Source: CAD feature listing. Evaluate the final solid. Frame: model axes, mm. A direction names the side the tool comes from. Give positions to 0.01 mm unless a question says otherwise; leave off trailing zeros. Order: outer loops, then holes, each group sorted by start corner. A loop starts at its lowest first (then second) coordinate and runs counter-clockwise, first axis right, second up. Notation, with made-up numbers: M 24.5,24 L 37.5,24 A32 ccw 37.5,58 Z; hole C -9.75,35 d9. An arc over 180 degrees is marked long. Answer as a JSON object with one key per item and string values. Group by question number.
1. Section query C-C (z = 40). Output: boundary loops of the cut face in (x, y).
2. Set-up query: faces 1 (the flat face through (-8, -0.5, 31)), 2 (the flat face through (-64, 6, 44.5)), 3 (the flat face through (-17, 3, 55)), 4 (the flat face through (-2, 3, 11.5)), 5 (the flat face through (-32.7, 7, 53)). Return all of +Z, -Z, +X, -X, +Y, -Y with unobstructed straight access to the full face (end or side cutting, diameter ignored); none if empty.
3. Section query A-A (x = -25.5). Output: boundary loops of the cut face in (y, z).
4. Section query B-B (x = -7). Output: boundary loops of the cut face in (y, z), plus the area to 4 significant figures.
5. Section query D-D (z = 58). Output: boundary loops of the cut face in (x, y).
6. Material intervals for L1, parallel to X at y = 1.1, z = 18; L2, parallel to Z at x = -80, y = 0.5; L3, parallel to Z at x = -85.5, y = 3.75, sorted ascending. Write a range as [from, to].
7. Pull-direction query (X, two-part tool) for faces 6 (the flat face through (-2, 3, 4)), 7 (the flat face through (-12.5, -1.5, 40)), 8 (the flat face through (-50, 4, 5)); classes: +X half, -X half, draft (parallel to the pull), parting line (faces both ways), or undercut.
8. Pin query (flat end, axial travel): P1, Ø3, axis at x = -47, z = 50, coming from the +Y side; P2, Ø5.5, axis at x = -64.5, y = 9.5, coming from the +Z side; P3, Ø1.5, axis at x = -26, y = 9.5, coming from the +Z side; P4, Ø4.5, axis at y = 3, z = 3, coming from the +X side. Return the tip coordinate at first contact, or that it passes through.
Autodesk Inventor part; units mm, degrees
ref_plane "YZ Plane" through (0, 0, 0) normal (1, 0, 0) x (0, 1, 0)
ref_plane "XZ Plane" through (0, 0, 0) normal (0, 1, 0) x (-1, 0, 0)
ref_plane "XY Plane" through (0, 0, 0) normal (0, 0, 1) x (1, 0, 0)
sketch "Skizze1" plane through (0, 0, 0) normal (0, 1, 0) x (-1, 0, 0)
  line L0 (0, 0) -> (85, 0)
  line L1 (85, 0) -> (85, 56)
  line L2 (85, 56) -> (0, 56)
  line L3 (0, 56) -> (0, 0)
  dimension "d0" = 85
  dimension "d1" = 56
extrude "Extrusion1" add sketch "Skizze1" along normal blind 1.5
sketch "Skizze2" plane through (0, 1.5, 0) normal (0, 1, 0) x (1, 0, 0)
  line L0 (0, 0) -> (-85, 0)
  line L1 (-86, -17.2) -> (-65, -17.2)
  line L2 (-65, -17.2) -> (-65, -1.2)
  line L3 (-65, -1.2) -> (-86, -1.2)
  line L4 (-86, -1.2) -> (-86, -17.2)
  line L5 (-85, 0) -> (-85, -56)
  dimension "d4" = 21
  dimension "d5" = 16
  dimension "d6" = 1.2
  dimension "d84" = 1
extrude "Extrusion2" add sketch "Skizze2" along normal blind 13.4
sketch "Skizze3" plane through (0, 1.5, 0) normal (0, 1, 0) x (1, 0, 0)
  line L0 (-85, -17.2) -> (-85, -56)
  line L1 (-92.7, -24) -> (-75.5, -24)
  line L2 (-75.5, -24) -> (-75.5, -37.2)
  line L3 (-75.5, -37.2) -> (-92.7, -37.2)
  line L4 (-92.7, -37.2) -> (-92.7, -24)
  line L5 (-85, -56) -> (0, -56)
  dimension "d9" = 7.7
  dimension "d10" = 17.2
  dimension "d11" = 13.2
  dimension "d85" = 18.8
extrude "Extrusion3" add sketch "Skizze3" along normal blind 16
sketch "Skizze4" plane through (0, 1.5, 0) normal (0, 1, 0) x (1, 0, 0)
  line L0 (0, 0) -> (-85, 0)
  line L1 (-65, -1.2) -> (-65, -17.2)
  line L2 (-50, 1) -> (-35, 1)
  line L3 (-35, 1) -> (-35, -10.8)
  line L4 (-35, -10.8) -> (-50, -10.8)
  line L5 (-50, -10.8) -> (-50, 1)
  dimension "d15" = 1
  dimension "d16" = 15
  dimension "d17" = 11.8
  dimension "d18" = 15
extrude "Extrusion4" add sketch "Skizze4" along normal blind 5.5
sketch "Skizze5" plane through (0, 1.5, 0) normal (0, 1, 0) x (1, 0, 0)
  line L0 (-85, -37.2) -> (-85, -56)
  line L1 (-85, -56) -> (0, -56)
  line L2 (-58.5, -44.5) -> (-70.5, -44.5)
  line L3 (-70.5, -44.5) -> (-70.5, -56)
  line L4 (-70.5, -56) -> (-58.5, -56)
  line L5 (-58.5, -56) -> (-58.5, -44.5)
  line L6 (-70.5, -56) -> (-58.5, -56)
  dimension "d21" = 11.5
  dimension "d22" = 12
  dimension "d23" = 14.5
extrude "Extrusion5" add sketch "Skizze5" along normal blind 10
sketch "Skizze6" plane through (-85, 0, 56) normal (0, 0, 1) x (1, 0, 0)
  line L0 (14.5, 11.5) -> (26.5, 11.5)
  circle A0 centre (20.5, 8) radius 3.5
  dimension "d26" = 7
  dimension "d27" = 3.5
extrude "Extrusion6" add sketch "Skizze6" along normal blind 3.5
sketch "Skizze7" plane through (0, 1.5, 0) normal (0, 1, 0) x (1, 0, 0)
  line L0 (-58.5, -44.5) -> (-58.5, -56)
  line L1 (-58.5, -56) -> (0, -56)
  line L2 (-51, -43.5) -> (-41, -43.5)
  line L3 (-41, -43.5) -> (-41, -53.5)
  line L4 (-41, -53.5) -> (-51, -53.5)
  line L5 (-51, -53.5) -> (-51, -43.5)
  dimension "d30" = 10
  dimension "d31" = 10
  dimension "d32" = 2.5
  dimension "d33" = 7.5
extrude "Extrusion7" add sketch "Skizze7" along normal blind 10.2
sketch "Skizze8" plane through (-51, 1.5, 53.5) normal (0, 0, 1) x (1, 0, 0)
  line L0 (0, 10.2) -> (10, 10.2)
  circle A0 centre (5, 6.2) radius 4
  point P0 (51, -1.5)
  dimension "d36" = 8
  dimension "d37" = 0
extrude "Extrusion8" add sketch "Skizze8" along normal blind 9
sketch "Skizze9" plane through (0, 1.5, 0) normal (0, 1, 0) x (1, 0, 0)
  line L0 (-58.5, -56) -> (0, -56)
  line L1 (0, -56) -> (0, 0)
  line L2 (-1, -55) -> (-33.7, -55)
  line L3 (-33.7, -55) -> (-33.7, -50)
  line L4 (-33.7, -50) -> (-1, -50)
  line L5 (-1, -50) -> (-1, -55)
  dimension "d40" = 32.7
  dimension "d41" = 5
  dimension "d42" = 1
  dimension "d43" = 1
extrude "Extrusion9" add sketch "Skizze9" along normal blind 2.5
sketch "Skizze10" plane through (0, 4, 0) normal (0, 1, 0) x (1, 0, 0)
  line L0 (-33.7, -55) -> (-1, -55)
  line L1 (-1, -55) -> (-1, -50)
  line L2 (-1, -50) -> (-33.7, -50)
  line L3 (-33.7, -50) -> (-33.7, -55)
  line L4 (-32.7, -51) -> (-2, -51)
  line L5 (-2, -51) -> (-2, -54)
  line L6 (-2, -54) -> (-32.7, -54)
  line L7 (-32.7, -54) -> (-32.7, -51)
  point P0 (0, 0)
  dimension "d50" = 1
  dimension "d51" = 1
  dimension "d52" = 1
  dimension "d53" = 1
extrude "Extrusion10" add sketch "Skizze10" along normal blind 6 contours L4 L5 L6 L7
sketch "Skizze11" plane through (0, 1.5, 0) normal (0, 1, 0) x (1, 0, 0)
  line L0 (0, -56) -> (0, 0)
  line L1 (0, 0) -> (-35, 0)
  line L2 (1, -4) -> (-4.6, -4)
  line L3 (-4.6, -4) -> (-4.6, -11.5)
  line L4 (-4.6, -11.5) -> (1, -11.5)
  line L5 (1, -11.5) -> (1, -4)
  dimension "d56" = 1
  dimension "d57" = 7.5
  dimension "d58" = 5.6
  dimension "d59" = 4
extrude "Extrusion11" add sketch "Skizze11" along normal blind 3
sketch "Skizze12" plane through (0, 0, 0) normal (0, -1, 0) x (1, 0, 0)
  line L0 (0, 0) -> (-85, 0)
  line L1 (0, 56) -> (0, 0)
  line L2 (-1, 43.5) -> (-18, 43.5)
  line L3 (-18, 43.5) -> (-18, 15.5)
  line L4 (-18, 15.5) -> (-1, 15.5)
  line L5 (-1, 15.5) -> (-1, 43.5)
  dimension "d62" = 15.5
  dimension "d63" = 17
  dimension "d64" = 28
  dimension "d65" = 1
extrude "Extrusion12" add sketch "Skizze12" along normal blind 0.5
sketch "Skizze13" plane through (0, -0.5, 0) normal (0, -1, 0) x (1, 0, 0)
  line L0 (-1, 43.5) -> (-18, 43.5)
  line L1 (-18, 43.5) -> (-18, 15.5)
  line L2 (-18, 15.5) -> (-1, 15.5)
  line L3 (-1, 15.5) -> (-1, 43.5)
  line L4 (-15, 42.5) -> (-1, 42.5)
  line L5 (-1, 42.5) -> (-1, 18.5)
  line L6 (-1, 18.5) -> (-15, 18.5)
  line L7 (-15, 18.5) -> (-15, 42.5)
  line L8 (-15, 37.5) -> (-10, 42.5)
  line L9 (-15, 37.5) -> (-7.9289, 37.5) construction
  point P0 (0, 0)
  dimension "d69" = 24
  dimension "d70" = 3
  dimension "d71" = 3
  dimension "d72" = 45
  dimension "d73" = 19
extrude "Extrusion13" add sketch "Skizze13" along normal blind 2 contours L3 L4 L7 L6 L2 L1 L0 | L8 L7 L4
sketch "Skizze14" plane through (0, 1.5, 0) normal (0, 1, 0) x (1, 0, 0)
  line L0 (0, 0) -> (-35, 0)
  line L1 (-85, -37.2) -> (-85, -56)
  line L2 (-85, -56) -> (-70.5, -56)
  line L3 (0, -56) -> (0, -11.5)
  circle A0 centre (-25.5, -18) radius 1.45
  circle A1 centre (-80, -43.5) radius 1.45
  dimension "d76" = 2.9
  dimension "d77" = 25.5
  dimension "d78" = 18
  dimension "d79" = 2.9
  dimension "d80" = 5
  dimension "d81" = 12.5
extrude "Extrusion14" cut sketch "Skizze14" against normal through all
properties part number "PCB"
Answer sheet:
{
 "1": {"outline": "M -85,0 L -18,0 L -18,-2.5 L -12.5,-2.5 L -12.5,-0.5 L -1,-0.5 L -1,0 L 0,0 L 0,1.5 L -85,1.5 Z"},
 "2": {"face 1": "+X, -Y", "face 2": "-X, +Y", "face 3": "+Z, +X, +Y", "face 4": "+X, +Y", "face 5": "+Z, -Z, +Y"},
 "3": {"outline": "M 0,0 L 1.5,0 L 1.5,16.55 L 0,16.55 Z; M 0,19.45 L 1.5,19.45 L 1.5,50 L 4,50 L 4,51 L 10,51 L 10,54 L 4,54 L 4,55 L 1.5,55 L 1.5,56 L 0,56 Z"},
 "4": {"outline": "M -2.5,15.5 L 0,15.5 L 0,0 L 1.5,0 L 1.5,50 L 4,50 L 4,51 L 10,51 L 10,54 L 4,54 L 4,55 L 1.5,55 L 1.5,56 L 0,56 L 0,43.5 L -2.5,43.5 L -2.5,42.5 L -0.5,42.5 L -0.5,18.5 L -2.5,18.5 Z", "area": "136.5 mm^2"},
 "5": {"outline": "C -64.5,8 d7; C -46,7.7 d8"},
 "6": {"L1": "[-85, -26.95], [-24.05, 0]", "L2": "[0, 42.05], [44.95, 56]", "L3": "[1.2, 17.2], [24, 37.2]"},
 "7": {"face 6": "draft", "face 7": "+X half", "face 8": "undercut"},
 "8": {"P1": "y = 11.7", "P2": "z = 59.5", "P3": "z = 54", "P4": "x = 1"}
}
